from build123d import *

# Parameters (mm, degrees)
F0_R     = 19
F1_DEPTH = 20
F2_R     = 3
F4_D     = 3
F4_DEPTH = 40
F4_TIP   = 0.9012909285
F6_D     = 3
F6_DEPTH = 40
F6_TIP   = 0.9012909285


with BuildPart() as f1:
    # F0 (on Top) → F1 (new body, symmetric)
    with BuildSketch(Plane.XY):
        Polygon((65.3352615237, 75.2357769758), (-54.6647384763, 75.2357769758), (-54.6647384763, 60.2357769758), (-54.6647384763, -9.7642230242), (-54.6647384763, -24.7642230242), (65.3352615237, -24.7642230242), align=None)
        with Locations((5.3352615237, 25.2357769758)):
            Circle(F0_R, mode=Mode.SUBTRACT)
    extrude(amount=F1_DEPTH, both=True)

    # F2
    f2_edges = [f1.edges().sort_by_distance(p)[0] for p in [
        (5.335262, 75.235777, 20),
        (-54.664738, 25.235777, 20),
        (5.335262, -24.764223, 20),
        (65.335262, 25.235777, 20),
        (-13.664738, 25.235777, 20),
        (65.335262, 25.235777, -20),
        (5.335262, 75.235777, -20),
        (-54.664738, 25.235777, -20),
        (5.335262, -24.764223, -20),
        (-13.664738, 25.235777, -20),
    ]]
    fillet(f2_edges, radius=F2_R)

    # F4
    with Locations(Plane(origin=(-54.6647384763, 0, 0), x_dir=(0, -1, 0), z_dir=(-1, 0, 0))):
        with Locations((9.7642230242, 0), (-60.2357769758, 0)):
            Hole(F4_D / 2, depth=F4_DEPTH)
            with Locations((0, 0, -(F4_DEPTH + F4_TIP / 2))):  # 118° drill point
                Cone(0, F4_D / 2, F4_TIP, mode=Mode.SUBTRACT)

    # F6
    with Locations(Plane.YZ.offset(65.3352615237)):
        with Locations((60.2357769758, 0), (-9.7642230242, 0)):
            Hole(F6_D / 2, depth=F6_DEPTH)
            with Locations((0, 0, -(F6_DEPTH + F6_TIP / 2))):  # 118° drill point
                Cone(0, F6_D / 2, F6_TIP, mode=Mode.SUBTRACT)


solid = f1.part
Input: part model. Units: mm. Frame: model coordinates. A direction names the side the tool comes from. Round coordinates to 2 decimals unless told otherwise and drop trailing zeros. Write each loop counter-clockwise with the first axis right and the second up, starting at its lowest first coordinate (ties: lowest second). Pieces come first, ordered by that corner, then holes.
1) Cut plane A-A (z = -15.5). Return the cut outline in (x, y), then the cut area to 3 significant figures.
2) Draft query along Y for faces 4 (the flat face through (65.335, 25, 0)), 5 (the conical face through (-13.92, -10.005, -0.1)), 6 (the flat face through (6, 75.236, 0)), 7 (the conical face through (-13.92, 59.99, 0.08)). Return one class per face: pulls with the +Y half, pulls with the -Y half, needs draft (parallel to the pull), parting line crosses it, or undercut.
3) Ray query, L1, parallel to Y at x = 39.5, z = 0; L2, parallel to X at y = 21, z = 14; L3, parallel to X at y = 15.5, z = -14.5. Return the intervals inside material, ascending.
4) Reachability of faces 1 (the cylindrical face through (45.055, 58.805, 0.451)), 2 (the cylindrical face through (-53.763, 24.536, 19.145)), 3 (the cylindrical face through (-34.385, -8.379, -0.575)) from +Z, -Z, +X, -X, +Y, -Y: full face, straight path, thin tool, end or side. Return the list, or none.
5) Contact query for a flat-ended pin moving along its axis: P1, Ø1.8, axis at y = 60.24, z = 0, coming from the +X side. Output: stop coordinate, or through.
Geometry says:
1. outline: (-54.66, -24.76) - (65.34, -24.76) - (65.34, 75.24) - (-54.66, 75.24) - close; hole circle Ø38 at (5.34, 25.24)
1. area: 10,900 mm2
2. face 4: needs draft
2. face 5: undercut
2. face 6: pulls with the +Y half
2. face 7: undercut
3. L1: y = -24.76 to -11.26, -8.26 to 58.74, 61.74 to 75.24
3. L2: x = -54.66 to -13.19, 23.86 to 65.34
3. L3: x = -54.66 to -10.98, 21.65 to 65.34
4. face 1: +X
4. face 2: +Z, -X, +Y, -Y
4. face 3: -X
5. P1: stops at x = 24.98
